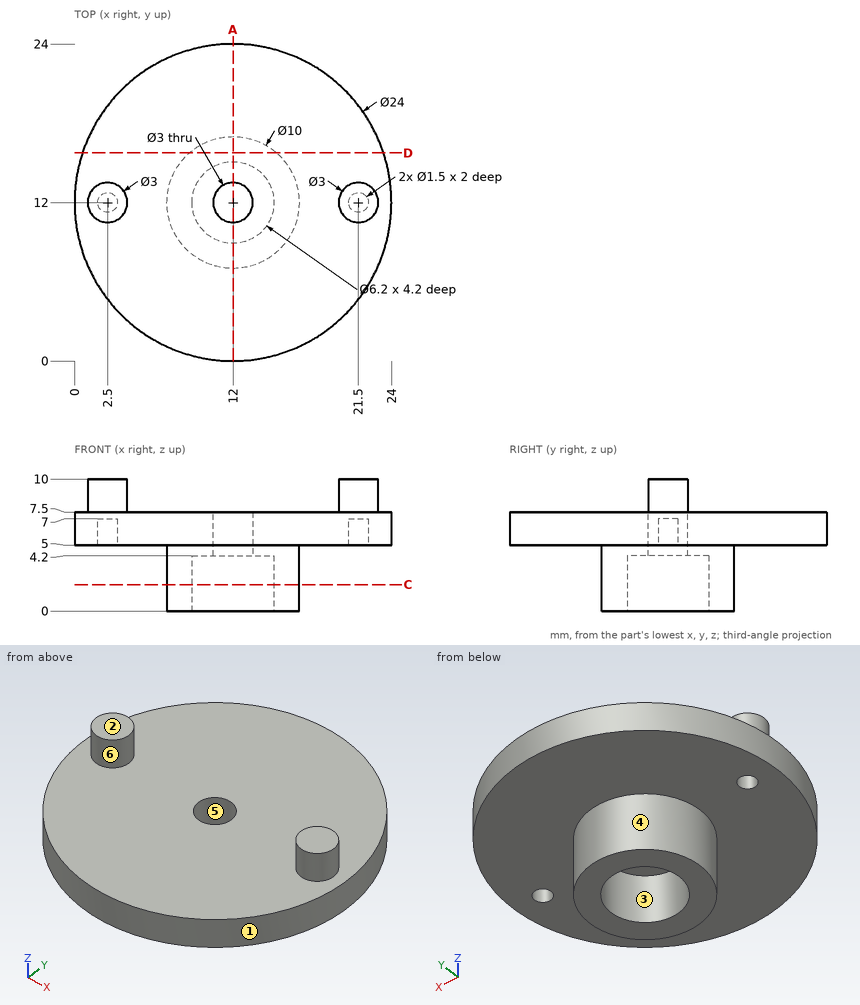
Can you work these out from the drawing? Everything is in mm from the part's minimum corner. A direction names the side the tool comes from. Give positions to 0.01 mm unless a question says otherwise; leave off trailing zeros. Loops run counter-clockwise (first coordinate to the right, second up) from the corner with the lowest first, then second, coordinate; pieces in that order, holes last. Notation, with made-up numbers: (-14.5, -16) -> (-7.5, -16) arc R24 ccw to (-7.5, 6) -> close; hole circle Ø7 at (62, -30.75). An arc over 180 degrees is marked (long way). Return JSON: item names as keys, results as strings.
Q1. I want a section at D-D, the plane y = 15.75. List the corners of the cut face in (x, z) for me, then the cut area to 3 significant figures.
Checks:
{"outline": "(0.6, 5) -> (8.69, 5) -> (8.69, 0) -> (15.31, 0) -> (15.31, 5) -> (23.4, 5) -> (23.4, 7.5) -> (0.6, 7.5) -> close", "area": "90.1 mm2"}
Q2. I need wall thicknesses on probe 1 along Y at (x, z) = (12, 5.7); probe 2 along Z at (x, y) = (9.25, 9.5); probe 3 along Z at (x, y) = (22, 11.5). Which ranges of each line are inside material? Lowest first, please.
Checks:
{"probe 1": "y = 0 to 10.5, 13.5 to 24", "probe 2": "z = 0 to 7.5", "probe 3": "z = 7 to 10"}
Q3. I want a section at C-C, the plane z = 2. List the corners of the cut face in (x, y) for me, then the cut area to 3 significant figures.
Checks:
{"outline": "circle Ø10 at (12, 12); hole circle Ø6.2 at (12, 12)", "area": "48.3 mm2"}
Q4. We'd pull the mould along X, two halves only. Please class the marked faces 1, 2 and 3: released by +X, released by -X, zero draft, split by the parting line, or undercut.
Checks:
{"face 1": "split by the parting line", "face 2": "zero draft", "face 3": "undercut"}
Q5. On a 3-axis mill with a long thin cutter (end or side, diameter ignored), from which of +Z, -Z, +X, -X, +Y, -Y can I reach the whole of each face in a straight line? I mean the marked faces 4, 5 and 6. Say none if no direction works.
Checks:
{"face 4": "-Z", "face 5": "+Z, -Z", "face 6": "+Z"}
Q6. For pin 1 Ø1.6 at (x, y) = (21.5, 12) entering from -Z; pin 2 Ø1.9 at (x, y) = (10.5, 11) entering from -Z; pin 3 Ø3 at (x, z) = (4.5, 8.5) entering from -Y, each with a flat end and sliding along its axis, tell me the tip position at first contact or that it passes through.
Checks:
{"pin 1": "stops at z = 5", "pin 2": "stops at z = 4.2", "pin 3": "stops at y = 1.84"}
Q7. I want a section at A-A, the plane x = 12. List the corners of the cut face in (y, z) for me.
Checks:
{"outline": "(0, 5) -> (7, 5) -> (7, 0) -> (8.9, 0) -> (8.9, 4.2) -> (10.5, 4.2) -> (10.5, 7.5) -> (0, 7.5) -> close; (13.5, 4.2) -> (15.1, 4.2) -> (15.1, 0) -> (17, 0) -> (17, 5) -> (24, 5) -> (24, 7.5) -> (13.5, 7.5) -> close"}
